from build123d import *

# Parameters (mm, degrees)
SKETCH_1_W          = 74
SKETCH_1_H          = 20
EXTRUDE_1_DEPTH     = 4
SKETCH_2_W          = 5
SKETCH_2_H          = 4
CUT_EXTRUDE_1_DEPTH = 5
FILLET_1_R          = 1


with BuildPart() as part:
    # 草图1 → 凸台-拉伸1 (new body)
    with BuildSketch(Plane.XY):
        with Locations((-37, 0)):
            Rectangle(SKETCH_1_W, SKETCH_1_H)
        with Locations((37, 0)):
            Rectangle(SKETCH_1_W, SKETCH_1_H)
    extrude(amount=EXTRUDE_1_DEPTH)

    # 草图2 → 切除-拉伸1 (cut)
    with BuildSketch(Plane.XY.offset(4)):
        with Locations((-67.5, -4)):
            Rectangle(SKETCH_2_W, SKETCH_2_H)
        with Locations((-67.5, 4)):
            Rectangle(SKETCH_2_W, SKETCH_2_H)
        with Locations((67.5, 4)):
            Rectangle(SKETCH_2_W, SKETCH_2_H)
        with Locations((67.5, -4)):
            Rectangle(SKETCH_2_W, SKETCH_2_H)
    extrude(amount=-CUT_EXTRUDE_1_DEPTH, mode=Mode.SUBTRACT)

    # 圆角1
    fillet_1_edges = [part.edges().sort_by_distance(p)[0] for p in [
        (-74, 0, 4),
        (74, 0, 4),
        (74, 0, 0),
        (-74, 0, 0),
        (74, 10, 2),
        (74, -10, 2),
        (-74, -10, 2),
        (-74, 10, 2),
    ]]
    fillet(fillet_1_edges, radius=FILLET_1_R)


solid = part.part
For this review, take the finished solid that the model builds, in its own axes (mm). A direction names the side the tool comes from. Give positions to 0.01 mm unless a question says otherwise; leave off trailing zeros. Loops run counter-clockwise (first coordinate to the right, second up) from the corner with the lowest first, then second, coordinate; pieces in that order, holes last.
Item 1: Take a section at B-B, the plane z = 2.2. State the section outline as (x, y) points.
Item 2: Draft analysis for pull direction Y (two halves, no side actions). For faces 1 (the flat face through (-1, -10, 2)), 2 (the flat face through (-70, 4, 2)), 3 (the flat face through (70, -4, 2)), 4 (the flat face through (-1, 0, 4)), state which applies: +Y half, -Y half, draft (parallel to the pull), parting line (faces both ways), or undercut.
Item 3: For line 1 along X through (y, z) = (-4.75, 2.45); line 2 along X through (y, z) = (3.25, 0.35); line 3 along X through (y, z) = (0.5, 0.9), list the stretches that pass through material, from the lowest coordinate up.
Item 4: Tool access review of faces 5 (the flat face through (-1, 0, 0)), 6 (the flat face through (-68, -6, 2)): name each direction out of +Z, -Z, +X, -X, +Y, -Y from which nothing blocks a thin tool from reaching the whole face with its end or side.
Item 5: Take a section at A-A, the plane y = 3.25. State the section outline as (x, z) points.
Calculated:
1. outline: (-74, -9) arc R1 ccw to (-73, -10) - (73, -10) arc R1 ccw to (74, -9) - (74, 9) arc R1 ccw to (73, 10) - (-73, 10) arc R1 ccw to (-74, 9) - close; hole (-70, -6) - (-65, -6) - (-65, -2) - (-70, -2) - close; hole (-70, 2) - (-65, 2) - (-65, 6) - (-70, 6) - close; hole (65, -6) - (70, -6) - (70, -2) - (65, -2) - close; hole (65, 2) - (70, 2) - (70, 6) - (65, 6) - close
2. face 1: -Y half
2. face 2: undercut
2. face 3: undercut
2. face 4: draft
3. line 1: x = -74 to -70, -65 to 65, 70 to 74
3. line 2: x = -73.76 to -70, -65 to 65, 70 to 73.76
3. line 3: x = -73.99 to 73.99
4. face 5: -Z, +X, -X, +Y, -Y
4. face 6: +Z, -Z
5. outline: (-74, 1) arc R1 ccw to (-73, 0) - (-70, 0) - (-70, 4) - (-73, 4) arc R1 ccw to (-74, 3) - close; (-65, 0) - (65, 0) - (65, 4) - (-65, 4) - close; (70, 0) - (73, 0) arc R1 ccw to (74, 1) - (74, 3) arc R1 ccw to (73, 4) - (70, 4) - close
